```python
from build123d import *

# Parameters (mm, degrees)
SKETCH2_W           = 40
SKETCH2_H           = 40
BOSS_EXTRUDE1_DEPTH = 4
SKETCH3_W           = 40
SKETCH3_H           = 10
BOSS_EXTRUDE2_DEPTH = 45
CUT_EXTRUDE1_REACH  = 68.312
SKETCH4_R           = 11
SKETCH4_R_2         = 2


with BuildPart() as part:
    # Sketch2 → Boss-Extrude1 (new body)
    with BuildSketch(Plane(origin=(0, 0, 0), x_dir=(1, 0, 0), z_dir=(0, 1, 0))):
        with Locations((7.772848934, 5.794927438)):
            Rectangle(SKETCH2_W, SKETCH2_H)
    extrude(amount=BOSS_EXTRUDE1_DEPTH)

    # Sketch3 → Boss-Extrude2 (add)
    with BuildSketch(Plane(origin=(0, 4, 0), x_dir=(1, 0, 0), z_dir=(0, 1, 0))):
        with Locations((7.772848934, -4.205072562)):
            Rectangle(SKETCH3_W, SKETCH3_H)
    extrude(amount=BOSS_EXTRUDE2_DEPTH)

    # Sketch4 → Cut-Extrude1 (cut, up to next)
    with BuildSketch(Plane.XY.offset(9.205072562), mode=Mode.PRIVATE) as cut_extrude1_sk1:
        with Locations((7.772848934, 27.5)):
            Circle(SKETCH4_R)
    cut_extrude1_tool1 = extrude(cut_extrude1_sk1.sketch, amount=-CUT_EXTRUDE1_REACH, mode=Mode.PRIVATE) & part.part
    # Sketch4 → Cut-Extrude1 (cut, up to next)
    with BuildSketch(Plane.XY.offset(9.205072562), mode=Mode.PRIVATE) as cut_extrude1_sk2:
        with Locations((19.897204587, 20.5)):
            Circle(SKETCH4_R_2)
    cut_extrude1_tool2 = extrude(cut_extrude1_sk2.sketch, amount=-CUT_EXTRUDE1_REACH, mode=Mode.PRIVATE) & part.part
    # Sketch4 → Cut-Extrude1 (cut, up to next)
    with BuildSketch(Plane.XY.offset(9.205072562), mode=Mode.PRIVATE) as cut_extrude1_sk3:
        with Locations((-4.351506719, 20.5)):
            Circle(SKETCH4_R_2)
    cut_extrude1_tool3 = extrude(cut_extrude1_sk3.sketch, amount=-CUT_EXTRUDE1_REACH, mode=Mode.PRIVATE) & part.part
    # Sketch4 → Cut-Extrude1 (cut, up to next)
    with BuildSketch(Plane.XY.offset(9.205072562), mode=Mode.PRIVATE) as cut_extrude1_sk4:
        with Locations((7.772848934, 41.5)):
            Circle(SKETCH4_R_2)
    cut_extrude1_tool4 = extrude(cut_extrude1_sk4.sketch, amount=-CUT_EXTRUDE1_REACH, mode=Mode.PRIVATE) & part.part
    add(cut_extrude1_tool1.solids().sort_by_distance((7.772849, 27.5, 9.205073))[0], mode=Mode.SUBTRACT)
    add(cut_extrude1_tool2.solids().sort_by_distance((19.897205, 20.5, 9.205073))[0], mode=Mode.SUBTRACT)
    add(cut_extrude1_tool3.solids().sort_by_distance((-4.351507, 20.5, 9.205073))[0], mode=Mode.SUBTRACT)
    add(cut_extrude1_tool4.solids().sort_by_distance((7.772849, 41.5, 9.205073))[0], mode=Mode.SUBTRACT)


solid = part.part
```
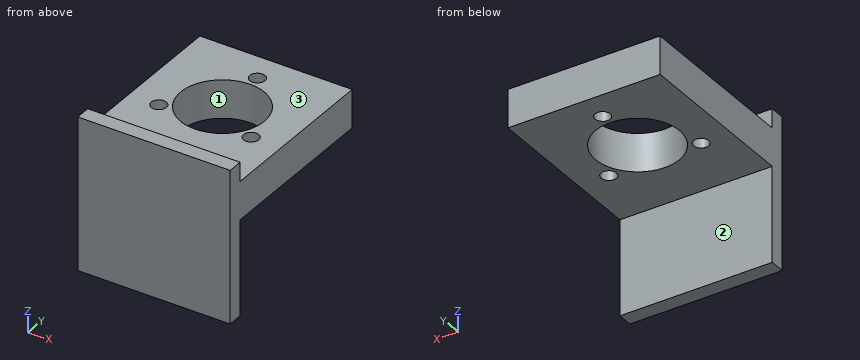
Design review of the part built by this model. Coordinates are the model's own, in mm. Face numbers are marked on the shaded views. A direction names the side the tool comes from. Give positions to 0.01 mm unless a question says otherwise; leave off trailing zeros. Write each loop counter-clockwise with the first axis right and the second up, starting at its lowest first coordinate (ties: lowest second). Pieces come first, ordered by that corner, then holes. Notation, with made-up numbers: (13, 2) -> (39, 2) arc R27 ccw to (39, 19) -> close; hole circle Ø5 at (-32, 59.5). An arc over 180 degrees is marked (long way). Answer in a Markdown table with one row per item.
(1) Clearance check with flat-ended pins moving along their axes: pin 1 (5 mm diameter, centred on x = -4.35, y = 20.5, fed in from -Z); pin 2 (20 mm diameter, centred on x = 7.77, y = 27.5, fed in from -Z); pin 3 (4 mm diameter, centred on x = 14.5, z = 11.5, fed in from +Y). State where each tip first meets the part, or that it passes through.
Results:
| item | result |
|---|---|
| pin 1 | z = -0.79 |
| pin 2 | through |
| pin 3 | y = 4 |
(2) To check wall thickness, follow probe 1 along X at (y, z) = (27, 7); probe 2 along Y at (x, z) = (18, -13.5); probe 3 along Z at (x, y) = (5, 43.5). State the ranges of each line that lie inside material, in increasing order.
Results:
| item | result |
|---|---|
| probe 1 | -12.23 to -3.22, 18.76 to 27.77 |
| probe 2 | 0 to 4 |
| probe 3 | -0.79 to 9.21 |
(3) Consider section D-D (x = 19.5). State the section outline as (y, z) points.
Results:
| item | result |
|---|---|
| outline | (0, -25.79) -> (4, -25.79) -> (4, -0.79) -> (18.54, -0.79) -> (18.54, 9.21) -> (4, 9.21) -> (4, 14.21) -> (0, 14.21) -> close; (22.46, -0.79) -> (49, -0.79) -> (49, 9.21) -> (22.46, 9.21) -> close |
(4) Consider section A-A (y = 41.5). State the section outline as (x, z) points, then the cut area to 3 significant figures.
Results:
| item | result |
|---|---|
| outline | (-12.23, -0.79) -> (5.77, -0.79) -> (5.77, 9.21) -> (-12.23, 9.21) -> close; (9.77, -0.79) -> (27.77, -0.79) -> (27.77, 9.21) -> (9.77, 9.21) -> close |
| area | 360 mm2 |
(5) Consider section C-C (y = 20.5). State the section outline as (x, z) points, then the cut area to 3 significant figures.
Results:
| item | result |
|---|---|
| outline | (-12.23, -0.79) -> (-6.35, -0.79) -> (-6.35, 9.21) -> (-12.23, 9.21) -> close; (-2.35, -0.79) -> (-0.71, -0.79) -> (-0.71, 9.21) -> (-2.35, 9.21) -> close; (16.26, -0.79) -> (17.9, -0.79) -> (17.9, 9.21) -> (16.26, 9.21) -> close; (21.9, -0.79) -> (27.77, -0.79) -> (27.77, 9.21) -> (21.9, 9.21) -> close |
| area | 150 mm2 |
(6) For the marked faces 1, 2 and 3, list the 3-axis set-ups (+Z, -Z, +X, -X, +Y, -Y) from which the entire face can be reached by the end or side of a thin tool; tool diameter is ignored.
Results:
| item | result |
|---|---|
| face 1 | +Z, -Z |
| face 2 | -Z, +X, -X, +Y |
| face 3 | +Z, +X, -X, +Y |
(7) Consider section B-B (x = -9). State the section outline as (y, z) points, then the cut area to 3 significant figures.
Results:
| item | result |
|---|---|
| outline | (0, -25.79) -> (4, -25.79) -> (4, -0.79) -> (49, -0.79) -> (49, 9.21) -> (4, 9.21) -> (4, 14.21) -> (0, 14.21) -> close |
| area | 610 mm2 |
